Autodesk Inventor part; units mm, degrees
ref_plane "YZ Plane" through (0, 0, 0) normal (1, 0, 0) x (0, 1, 0)
ref_plane "XZ Plane" through (0, 0, 0) normal (0, 1, 0) x (-1, 0, 0)
ref_plane "XY Plane" through (0, 0, 0) normal (0, 0, 1) x (1, 0, 0)
sketch "Sketch1" plane through (0, 0, 0) normal (1, 0, 0) x (0, 1, 0)
  line L0 (-0.5, 0) -> (0.55, 0)
  line L1 (3.0679, 1.692) -> (-10.4321, 1.692)
  line L2 (-10.4321, 1.692) -> (-10.4321, 4.692)
  line L3 (-10.4321, 4.692) -> (3.0679, 4.692)
  line L4 (3.0679, 4.692) -> (3.0679, 1.692)
  line L5 (-0.9321, 1.692) -> (-6.4321, 1.692)
  line L6 (-6.4321, 1.692) -> (-6.4321, 2.692)
  line L7 (-6.4321, 2.692) -> (-0.9321, 2.692)
  line L8 (-0.9321, 2.692) -> (-0.9321, 1.692)
  line L9 (-3.6821, 1.692) -> (-3.6821, 4.692) construction
  line L10 (1.0679, 4.692) -> (1.0679, 1.692) construction
  line L11 (-0.5, 0) -> (0.55, 0) construction
  point P0 (0, 0)
  dimension "d0" = 5.5
  dimension "d1" = 4
  dimension "d2" = 2
  dimension "d3" = 1
  dimension "d4" = 2
extrude "Extrusion1" add sketch "Sketch1" along normal blind 6 contours L1 L8 L7 L6 L2 L3 L4
sketch "Sketch2" plane through (0, -10.4321, 4.692) normal (0, 0, 1) x (1, 0, 0)
  line L0 (0, 11.5) -> (6, 11.5) construction
  line L1 (6, 13.5) -> (6, 0) construction
  point P0 (0, 10.4321)
  point P1 (3, 11.5)
hole "Hole1" at (3, 1.0679, 4.692) direction (0, 0, -1) diameter 2.1 end through all
ref_plane "Work Plane1" through (0, -3.6821, 4.692) normal (0, 1, 0) x (1, 0, 0)
mirror "Mirror1" about plane through (0, -3.6821, 4.692) normal (0, 1, 0) of "Hole1"
properties part number "Encoder_Cable_Clamp"
CAD build for the part. Positions are in the model's coordinates, mm. A direction names the side the tool comes from. Round coordinates to 2 decimals unless told otherwise and drop trailing zeros. Loops run counter-clockwise (first coordinate to the right, second up) from the corner with the lowest first, then second, coordinate; pieces in that order, holes last. Notation, with made-up numbers: (80, -15.75) - (118, -15.75) arc R30 cw to (118, 18.25) - close; hole circle Ø11 at (60, 85.5). An arc over 180 degrees is marked (long way). Put each result on its own line as item: value.
1. Slice it at D-D on y = 0.5. List the corners of the cut face in (x, z), and give its area (3 significant figures).
Geometry check:
outline: (0, 1.69) - (2.12, 1.69) - (2.12, 4.69) - (0, 4.69) - close; (3.88, 1.69) - (6, 1.69) - (6, 4.69) - (3.88, 4.69) - close
area: 12.7 mm²
2. Two-plate mould, pull along Y, no slides. Class faces 1 (the cylindrical face through (3.32, -7.43, 3.17)), 2 (the flat face through (3, -4, 2.692)), 3 (the flat face through (6, -4, 3)), 4 (the flat face through (3, -10.432, 3)): released by +Y, released by -Y, zero draft, split by the parting line, or undercut.
Geometry check:
face 1: undercut
face 2: undercut
face 3: zero draft
face 4: released by -Y
3. 3-axis set-ups, long thin cutter, end or side, ignore diameter. For faces 5 (the flat face through (1.6, -8.4, 1.692)), 6 (the flat face through (3, -0.932, 2)): which of +Z, -Z, +X, -X, +Y, -Y reach the whole face in a straight line?
Geometry check:
face 5: -Z, +X, -X, +Y, -Y
face 6: -Z, +X, -X
4. Slice it at C-C on x = 5.5. List the corners of the cut face in (y, z), and give its area (3 significant figures).
Geometry check:
outline: (-10.43, 1.69) - (-6.43, 1.69) - (-6.43, 2.69) - (-0.93, 2.69) - (-0.93, 1.69) - (3.07, 1.69) - (3.07, 4.69) - (-10.43, 4.69) - close
area: 35.0 mm²
5. Wall check: line 1 (Y direction, x = 3, z = 3.1); line 2 (Y direction, x = 3.4, z = 4.1); line 3 (Y direction, x = 5.25, z = 2.4). Give the ranges that are in metal, low to high.
Geometry check:
line 1: -10.43 to -9.48, -7.38 to 0.02, 2.12 to 3.07
line 2: -10.43 to -9.4, -7.46 to 0.1, 2.04 to 3.07
line 3: -10.43 to -6.43, -0.93 to 3.07
6. Slice it at A-A on z = 2.55. List the corners of the cut face in (x, y), and give its area (3 significant figures).
Geometry check:
outline: (0, -10.43) - (6, -10.43) - (6, -6.43) - (0, -6.43) - close; (0, -0.93) - (6, -0.93) - (6, 3.07) - (0, 3.07) - close; hole circle Ø2.1 at (3, -8.43); hole circle Ø2.1 at (3, 1.07)
area: 41.1 mm²
7. Slice it at B-B on x = 3. List the corners of the cut face in (y, z), and give its area (3 significant figures).
Geometry check:
outline: (-10.43, 1.69) - (-9.48, 1.69) - (-9.48, 4.69) - (-10.43, 4.69) - close; (-7.38, 1.69) - (-6.43, 1.69) - (-6.43, 2.69) - (-0.93, 2.69) - (-0.93, 1.69) - (0.02, 1.69) - (0.02, 4.69) - (-7.38, 4.69) - close; (2.12, 1.69) - (3.07, 1.69) - (3.07, 4.69) - (2.12, 4.69) - close
area: 22.4 mm²
8. Pin check, flat tips, straight feed: P1, Ø1.3, axis at x = 3, y = -8.43, coming from the -Z side; P2, Ø3, axis at x = 3, y = -4, coming from the -Z side. Stop position of each tip, or through.
Geometry check:
P1: through
P2: z = 2.69
